Autodesk Inventor part; units mm, degrees
ref_plane "YZ Plane" through (0, 0, 0) normal (1, 0, 0) x (0, 1, 0)
ref_plane "XZ Plane" through (0, 0, 0) normal (0, 1, 0) x (-1, 0, 0)
ref_plane "XY Plane" through (0, 0, 0) normal (0, 0, 1) x (1, 0, 0)
sketch "Sketch1" plane through (0, 0, 0) normal (0, 1, 0) x (-1, 0, 0)
  circle A0 centre (0, 0) radius 3.45
  line L0 (0, 0) -> (-13.55, 0) construction
  line L1 (-0.0814, 2.4486) -> (-13.6164, 1.9989)
  line L2 (-13.6164, -1.9989) -> (-0.0814, -2.4486)
  arc A1 (-0.0814, -2.4486) -> (-0.0814, 2.4486) centre (0, 0) ccw
  arc A2 (-13.6164, 1.9989) -> (-13.6164, -1.9989) centre (-13.55, 0) ccw
  point P0 (-6.775, 0)
  point P1 (-15.55, 0)
  point P2 (3.45, 0)
  dimension "d0" = 6.9
  dimension "d2" = 4
  dimension "d3" = 1
  dimension "d4" = 19
extrude "Extrusion1" add sketch "Sketch1" along normal blind 1.4
extrude "Extrusion2" add sketch "Sketch1" along normal blind 3.7 contours A0 L2 A1 L1 | L1 A1 L2 A0
sketch "Sketch2" plane through (0, 3.7, 0) normal (0, 1, 0) x (1, 0, 0)
  circle A0 centre (0, 0) radius 3.45 construction
  circle A1 centre (0, 0) radius 1.2
  dimension "d9" = 2.4
extrude "Extrusion3" cut sketch "Sketch2" against normal through all
sketch "Sketch3" plane through (0, 3.7, 0) normal (0, 1, 0) x (1, 0, 0)
  circle A0 centre (0, 0) radius 3.45 construction
  circle A1 centre (0, 0) radius 2.3
  dimension "d12" = 4.6
extrude "Extrusion4" cut sketch "Sketch3" against normal blind 2
sketch "Sketch4" plane through (0, 0, 0) normal (0, -1, 0) x (1, 0, 0)
  arc A0 (2.509, 2.368) -> (2.509, -2.368) centre (0, 0) ccw construction
  circle A1 centre (0, 0) radius 2.35
  dimension "d15" = 1.1
extrude "Extrusion5" cut sketch "Sketch4" against normal blind 1
sketch "Sketch5" plane through (0, 0, 0) normal (0, -1, 0) x (1, 0, 0)
  arc A0 (13.6164, -1.9989) -> (13.6164, 1.9989) centre (13.55, 0) ccw construction
  line L0 (13.55, 0) -> (10.05, 0)
  line L1 (10.05, 0) -> (6.55, 0)
  line L2 (6.55, 0) -> (3.05, 0)
  point P0 (8.3, 0)
  point P1 (4.8, 0)
  point P2 (11.8, 0)
  point P3 (4.8, 0)
  dimension "d18" = 3.5
hole "Hole1" at (13.55, 0, 0) at (10.05, 0, 0) at (8.3, 0, 0) at (6.55, 0, 0) at (4.8, 0, 0) at (11.8, 0, 0) direction (0, 1, 0) diameter 0.3 end through all
properties part number "SG90Horn1" material "PC/ABS Plastic"
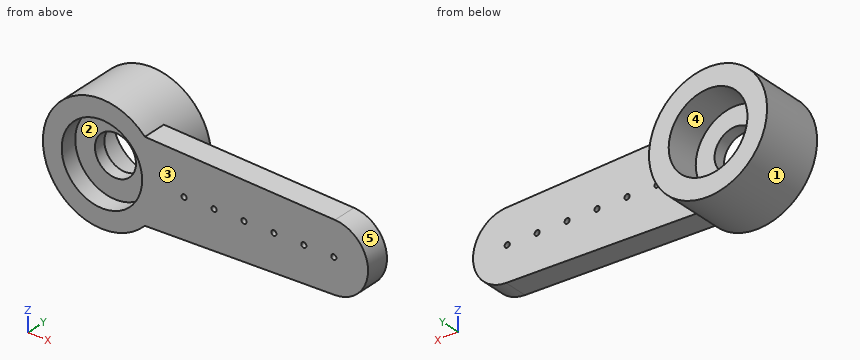
The listing builds one solid part. Answer for the finished solid, in the listing's coordinates (mm). Face numbers are marked on the shaded views. A direction names the side the tool comes from. Give positions to 0.01 mm unless a question says otherwise; leave off trailing zeros. Loops run counter-clockwise (first coordinate to the right, second up) from the corner with the lowest first, then second, coordinate; pieces in that order, holes last. Notation, with made-up numbers: M -28.75,-39 L 29.25,-39 A20 cw 29.25,-25 Z; hole C 79,-29 d11. An arc over 180 degrees is marked long. One line per item, written item: value.
Q1. Flat-ended cylindrical pins translate along their axes: P1, Ø2, axis at x = 13.5, y = 1, coming from the +Z side; P2, Ø4, axis at x = 9.5, z = 0, coming from the -Y side; P3, Ø4, axis at x = 0, z = 0, coming from the -Y side; P4, Ø2, axis at x = 2.5, y = 1, coming from the -Z side. Find the tip coordinate at first contact, or state that the pin passes through.
Working result:
P1: stops at z = 2.04
P2: stops at y = 0
P3: stops at y = 1
P4: stops at z = -3.11
Q2. For the marked faces 4 and 5, determine the directions among +Z, -Z, +X, -X, +Y, -Y from which every point of the face is accessible in a straight line to the end or side of a thin tool.
Working result:
face 4: +Y
face 5: +X, +Y, -Y
Q3. A cutting plane is placed at A-A on y = 0.6. Determine the outline of the cut face in (x, z), then the cut area to 3 significant figures.
Working result:
outline: M 2.51,-2.37 L 13.62,-2 A2 ccw 13.62,2 L 2.51,2.37 A3.45 ccw long Z; hole C 0,0 d4.7; hole C 4.8,0 d0.3; hole C 6.55,0 d0.3; hole C 8.3,0 d0.3; hole C 10.05,0 d0.3; hole C 11.8,0 d0.3; hole C 13.55,0 d0.3
area: 71.1 mm^2
Q4. Determine the mould class of the marked faces 1, 2 and 3 for opening direction Z: +Z half, -Z half, draft (parallel to the pull), parting line (faces both ways), or undercut.
Working result:
face 1: parting line
face 2: undercut
face 3: draft
Q5. A cutting plane is placed at B-B on z = -1. Determine the outline of the cut face in (x, y).
Working result:
outline: M -3.3,0 L -2.13,0 L -2.13,1 L -0.66,1 L -0.66,1.7 L -2.07,1.7 L -2.07,3.7 L -3.3,3.7 Z; M 0.66,1 L 2.13,1 L 2.13,0 L 15.28,0 L 15.28,1.4 L 3.3,1.4 L 3.3,3.7 L 2.07,3.7 L 2.07,1.7 L 0.66,1.7 Z
Q6. Find the intervals of material crossed by line 1 (Z direction, x = 0, y = 0.4); line 2 (X direction, y = 3.3, z = 0); line 3 (Z direction, x = 0, y = 1.5), in increasing order. Write a range as from..to.
Working result:
line 1: z = -3.45..-2.35, 2.35..3.45
line 2: x = -3.45..-2.3, 2.3..3.45
line 3: z = -3.45..-1.2, 1.2..3.45
Q7. A cutting plane is placed at D-D on y = 3.35. Determine the outline of the cut face in (x, z).
Working result:
outline: C 0,0 d6.9; hole C 0,0 d4.6
